Autodesk Inventor part; units mm, degrees
ref_plane "YZ Plane" through (0, 0, 0) normal (1, 0, 0) x (0, 1, 0)
ref_plane "XZ Plane" through (0, 0, 0) normal (0, 1, 0) x (-1, 0, 0)
ref_plane "XY Plane" through (0, 0, 0) normal (0, 0, 1) x (1, 0, 0)
sketch "Sketch3" plane through (0, 0, 0) normal (0, 0, 1) x (1, 0, 0)
  line L0 (0, 0) -> (300, 0)
  line L1 (300, 0) -> (300, 30)
  line L2 (300, 30) -> (-5.542, 53.9641)
  line L3 (45, 50) -> (45, 0)
  dimension "d11" = 300
  dimension "d12" = 30
  dimension "d13" = 45
  dimension "d14" = 50
extrude "Plate1" add sketch "Sketch3" along normal mid plane 10
fillet "Corner Round1" radius 6 1 edges at (300, 30, 0)
equation "\"d15\" = Thickness"
equation "\"BendReliefDepth\" = 0.5 * Thickness"
properties part number "PRS 1614 charging hatch reinf 500mm" material "Steel"
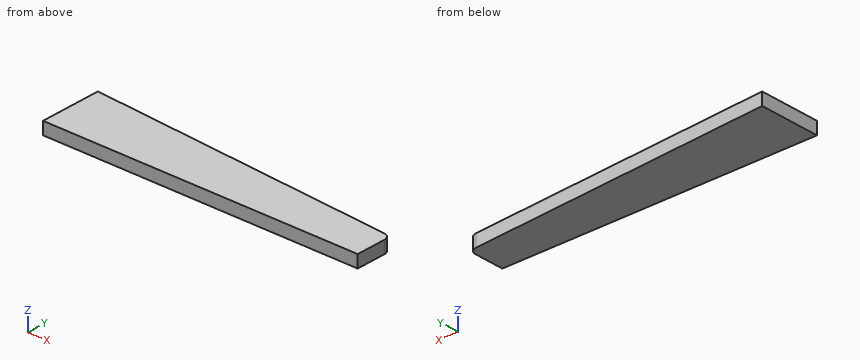
Geometry check sheet. Reference: the model listing, model coordinates, mm. Round coordinates to 2 decimals unless told otherwise and drop trailing zeros. Loops run counter-clockwise (first coordinate to the right, second up) from the corner with the lowest first, then second, coordinate; pieces in that order, holes last.
Item 1: Thickness scan on line 1 (Y direction, x = 222.5, z = -3.25); line 2 (X direction, y = 28.5, z = 1.75); line 3 (Y direction, x = 289, z = 3.25). Record the ranges inside material, lowest first.
Item 2: Cross-section at A-A on z = 3. Record the boundary of the cut face in (x, y), then the cut area to 3 significant figures.
Item 3: Cross-section at C-C on y = 46.5. Record the boundary of the cut face in (x, z), then the cut area to 3 significant figures.
Item 4: Gauge pin test, flat ends, axial feed: pin 1 (2 mm diameter, centred on x = 218.5, z = -1, fed in from +Y); pin 2 (6 mm diameter, centred on x = 218, z = 2, fed in from +Y). Record the tip position at first contact, or that the pin passes through.
Item 5: Cross-section at B-B on x = 282. Record the boundary of the cut face in (y, z), then the cut area to 3 significant figures.
Answer sheet:
1. line 1: y = 0 to 36.08
1. line 2: x = 45 to 298.43
1. line 3: y = 0 to 30.86
2. outline: (45, 0) - (300, 0) - (300, 24.45) arc R6 ccw to (294.47, 30.43) - (45, 50) - close
2. area: 10,200 mm2
3. outline: (45, -5) - (89.63, -5) - (89.63, 5) - (45, 5) - close
3. area: 446 mm2
4. pin 1: stops at y = 36.47
4. pin 2: stops at y = 36.67
5. outline: (0, -5) - (31.41, -5) - (31.41, 5) - (0, 5) - close
5. area: 314 mm2
